from build123d import *

# Parameters (mm, degrees)
SKETCH1_R           = 31.75
BOSS_EXTRUDE1_DEPTH = 4.7625
CUT_EXTRUDE1_REACH  = 47.153
CUT_EXTRUDE2_REACH  = 46.61


with BuildPart() as part:
    # Sketch1 → Boss-Extrude1 (new body)
    with BuildSketch(Plane(origin=(0, 0, 0), x_dir=(1, 0, 0), z_dir=(0, 1, 0))):
        with Locations(Location((0, 0, 0), (0, 0, 90))):
            Circle(SKETCH1_R)
    extrude(amount=BOSS_EXTRUDE1_DEPTH)

    # Sketch2 → Cut-Extrude1 (cut, up to next)
    with BuildSketch(Plane(origin=(0, 4.7625, 0), x_dir=(1, 0, 0), z_dir=(0, 1, 0)), mode=Mode.PRIVATE) as cut_extrude1_sk1:
        with BuildLine():
            Line((-6.985, -30.972120932), (-6.985, -25.892120932))
            Line((-6.985, -25.892120932), (6.985, -25.892120932))
            Line((6.985, -25.892120932), (6.985, -30.972120932))
            ThreePointArc((6.985, -30.972120932), (0, -31.75), (-6.985, -30.972120932))
        make_face()
    cut_extrude1_tool1 = extrude(cut_extrude1_sk1.sketch, amount=-CUT_EXTRUDE1_REACH, mode=Mode.PRIVATE) & part.part
    # Sketch2 → Cut-Extrude1 (cut, up to next)
    with BuildSketch(Plane(origin=(0, 4.7625, 0), x_dir=(1, 0, 0), z_dir=(0, 1, 0)), mode=Mode.PRIVATE) as cut_extrude1_sk2:
        with BuildLine():
            Line((-6.985, 30.972120932), (-6.985, 25.892120932))
            Line((-6.985, 25.892120932), (6.985, 25.892120932))
            Line((6.985, 25.892120932), (6.985, 30.972120932))
            ThreePointArc((6.985, 30.972120932), (0, 31.75), (-6.985, 30.972120932))
        make_face()
    cut_extrude1_tool2 = extrude(cut_extrude1_sk2.sketch, amount=-CUT_EXTRUDE1_REACH, mode=Mode.PRIVATE) & part.part
    add(cut_extrude1_tool1.solids().sort_by_distance((0, 4.7625, 28.696841))[0], mode=Mode.SUBTRACT)
    add(cut_extrude1_tool2.solids().sort_by_distance((0, 4.7625, -28.696841))[0], mode=Mode.SUBTRACT)

    # Sketch3 → Cut-Extrude2 (cut, up to next)
    with BuildSketch(Plane(origin=(0, 4.7625, 0), x_dir=(1, 0, 0), z_dir=(0, 1, 0)), mode=Mode.PRIVATE) as cut_extrude2_sk1:
        with BuildLine():
            Line((18.930734485, -18.995247911), (25.915734485, -6.89687302))
            Line((25.915734485, -6.89687302), (30.315143536, -9.43687302))
            ThreePointArc((30.315143536, -9.43687302), (27.49630657, -15.875), (23.330143536, -21.535247911))
            Line((23.330143536, -21.535247911), (18.930734485, -18.995247911))
        make_face()
    cut_extrude2_tool1 = extrude(cut_extrude2_sk1.sketch, amount=-CUT_EXTRUDE2_REACH, mode=Mode.PRIVATE) & part.part
    # Sketch3 → Cut-Extrude2 (cut, up to next)
    with BuildSketch(Plane(origin=(0, 4.7625, 0), x_dir=(1, 0, 0), z_dir=(0, 1, 0)), mode=Mode.PRIVATE) as cut_extrude2_sk2:
        with BuildLine():
            Line((-25.915734485, 6.89687302), (-30.315143536, 9.43687302))
            ThreePointArc((-30.315143536, 9.43687302), (-27.49630657, 15.875), (-23.330143536, 21.535247911))
            Line((-23.330143536, 21.535247911), (-18.930734485, 18.995247911))
            Line((-18.930734485, 18.995247911), (-25.915734485, 6.89687302))
        make_face()
    cut_extrude2_tool2 = extrude(cut_extrude2_sk2.sketch, amount=-CUT_EXTRUDE2_REACH, mode=Mode.PRIVATE) & part.part
    add(cut_extrude2_tool1.solids().sort_by_distance((24.852194, 4.7625, 14.348421))[0], mode=Mode.SUBTRACT)
    add(cut_extrude2_tool2.solids().sort_by_distance((-24.852194, 4.7625, -14.348421))[0], mode=Mode.SUBTRACT)


solid = part.part
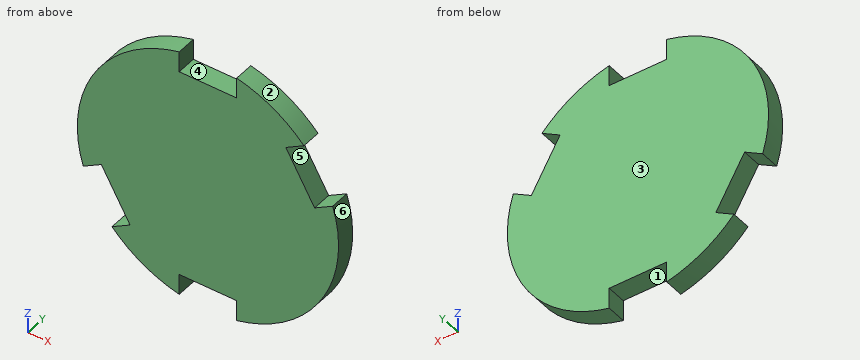
CAD build for the part. Positions are in the model's coordinates, mm. Face numbers are marked on the shaded views. A direction names the side the tool comes from. Give positions to 0.01 mm unless a question says otherwise; leave off trailing zeros. Write each loop counter-clockwise with the first axis right and the second up, starting at its lowest first coordinate (ties: lowest second). Pieces come first, ordered by that corner, then holes. Notation, with made-up numbers: M 12,-9.75 L 66,-9.75 A14 cw 66,-2.75 Z; hole C 75,44 d4. An arc over 180 degrees is marked long. Put each result on its own line as item: value. Start each with the question number.
(1) Probe L1, parallel to Z at x = 19, y = 3.4; L2, parallel to Z at x = 1.5, y = 2.7; L3, parallel to X at y = 1.25, z = 27.5 (3 decimals). List the from-to ranges inside material, lowest first.
(2) Mould opens along X. For the marked faces 1, 2 and 3 say: +X half, -X half, draft (parallel to the pull), parting line (faces both ways), or undercut.
(3) Band-saw the part on A-A, the plane y = 1.85. Write the cut outline in (x, z) (3 decimals), and give its area (3 significant figures).
(4) Flat gauge pins, fed straight in: pin 1 Ø2.5 at (y, z) = (2.5, 27.5) entering from +X; pin 2 Ø2 at (y, z) = (3.5, 12.5) entering from -X; pin 3 Ø1.4 at (x, y) = (0, 1.5) entering from +Z. Where does each tip first touch, or does it go through?
(5) Band-saw the part on B-B, the plane x = 20. Write the cut outline in (y, z).
(6) Band-saw the part on C-C, the plane z = 20. Write the cut outline in (x, y).
(7) Band-saw the part on D-D, the plane x = -3.5. Write the cut outline in (y, z), and give its area (3 significant figures).
(8) Which spindle directions (+Z, -Z, +X, -X, +Y, -Y) get a long thin tool onto all of the face, cutting with end or side? Do the marked faces 4, 5 and 6. Say none if no direction does.
Response values:
1. L1: z = -25.44 to 18.88, 19.04 to 25.44
1. L2: z = -25.89 to 25.89
1. L3: x = -15.869 to -6.985, 6.985 to 15.869
2. face 1: undercut
2. face 2: +X half
2. face 3: draft
3. outline: M -30.315,-9.437 L -25.916,-6.897 L -18.931,-18.995 L -23.33,-21.535 A31.75 ccw -6.985,-30.972 L -6.985,-25.892 L 6.985,-25.892 L 6.985,-30.972 A31.75 ccw 30.315,9.437 L 25.916,6.897 L 18.931,18.995 L 23.33,21.535 A31.75 ccw 6.985,30.972 L 6.985,25.892 L -6.985,25.892 L -6.985,30.972 A31.75 ccw Z
3. area: 2,850 mm2
4. pin 1: stops at x = 17.86
4. pin 2: stops at x = -29.59
4. pin 3: stops at z = 25.89
5. outline: M 0,-24.66 L 4.76,-24.66 L 4.76,17.14 L 0,17.14 Z; M 0,19.61 L 4.76,19.61 L 4.76,24.66 L 0,24.66 Z
6. outline: M -24.66,0 L 20.67,0 L 20.67,4.76 L -24.66,4.76 Z
7. outline: M 0,-25.89 L 4.76,-25.89 L 4.76,25.89 L 0,25.89 Z
7. area: 247 mm2
8. face 4: +Z, +Y, -Y
8. face 5: +Y, -Y
8. face 6: +X, +Y, -Y
